Can you work these out from the model? Positions are in its coordinate system, mm. Face numbers are marked on the shaded views. A direction names the side the tool comes from. Give positions to 0.01 mm unless a question says otherwise; leave off trailing zeros. Loops run counter-clockwise (first coordinate to the right, second up) from the corner with the lowest first, then second, coordinate; pieces in that order, holes last. Notation, with made-up numbers: M 65.25,62 L 108.25,62 A29 cw 108.25,85 Z; hole C -22.75,20.25 d11. An arc over 180 degrees is marked long. Answer as a JSON object with one key per item and string values.
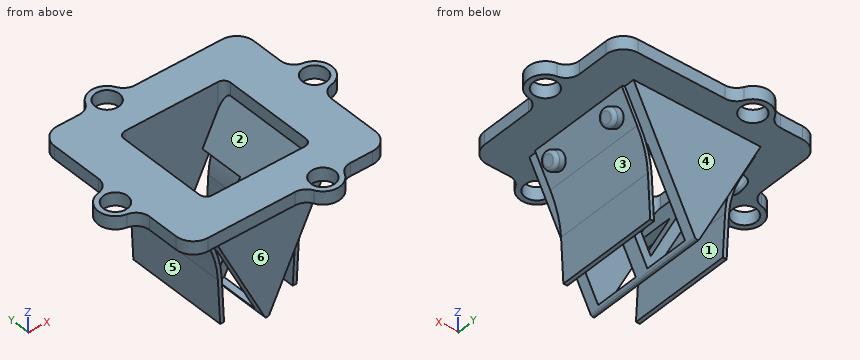
```python
from build123d import *

# Parameters (mm, degrees)
SKETCH_1_R          = 3.5
EXTRUDE_1_DEPTH     = 3.8
LOFT_START          = -18
LOFT_1_DEPTH        = 36
FILLET_1_R          = 0.5
CUT_EXTRUDE_1_DEPTH = 15
FILLET_2_R          = 2
SKETCH_6_W          = 22
SKETCH_6_H          = 13
CUT_EXTRUDE_2_DEPTH = 19
EXTRUDE_2_DEPTH     = 15
SKETCH_8_R          = 2.5
EXTRUDE_3_DEPTH     = 3
FILLET_5_R          = 1
SKETCH_9_R          = 2.5
EXTRUDE_4_DEPTH     = 3
FILLET_6_R          = 1


# Read off the part's stored shape, not the designer's step: По сечениям1
with BuildPart() as part:
    # Эскиз1 → Бобышка-Вытянуть1 (new body)
    with BuildSketch(Plane.XY):
        with BuildLine():
            Line((-24, -26), (1.437742252, -26))
            ThreePointArc((1.437742252, -26), (3.545927358, -26.600653658), (5.020967918, -28.222222222))
            ThreePointArc((5.020967918, -28.222222222), (9.5, -31), (13.979032082, -28.222222222))
            ThreePointArc((13.979032082, -28.222222222), (15.454072642, -26.600653658), (17.562257748, -26))
            Line((17.562257748, -26), (24, -26))
            ThreePointArc((24, -26), (27.535533906, -24.535533906), (29, -21))
            Line((29, -21), (29, -5.874119675))
            ThreePointArc((29, -5.874119675), (29.944949537, -3.292130777), (32.333333333, -1.930066486))
            ThreePointArc((32.333333333, -1.930066486), (36.5, 3), (32.333333333, 7.930066486))
            ThreePointArc((32.333333333, 7.930066486), (29.944949537, 9.292130777), (29, 11.874119675))
            Line((29, 11.874119675), (29, 21))
            ThreePointArc((29, 21), (27.535533906, 24.535533906), (24, 26))
            Line((24, 26), (-1.437742252, 26))
            ThreePointArc((-1.437742252, 26), (-3.545927358, 26.600653658), (-5.020967918, 28.222222222))
            ThreePointArc((-5.020967918, 28.222222222), (-9.5, 31), (-13.979032082, 28.222222222))
            ThreePointArc((-13.979032082, 28.222222222), (-15.454072642, 26.600653658), (-17.562257748, 26))
            Line((-17.562257748, 26), (-24, 26))
            ThreePointArc((-24, 26), (-27.535533906, 24.535533906), (-29, 21))
            Line((-29, 21), (-29, 5.874119675))
            ThreePointArc((-29, 5.874119675), (-29.944949537, 3.292130777), (-32.333333333, 1.930066486))
            ThreePointArc((-32.333333333, 1.930066486), (-36.5, -3), (-32.333333333, -7.930066486))
            ThreePointArc((-32.333333333, -7.930066486), (-29.944949537, -9.292130777), (-29, -11.874119675))
            Line((-29, -11.874119675), (-29, -21))
            ThreePointArc((-29, -21), (-27.535533906, -24.535533906), (-24, -26))
        make_face()
        with Locations(Location((31.5, 3, 0), (0, 0, 180))):
            Circle(SKETCH_1_R, mode=Mode.SUBTRACT)
        with Locations(Location((-9.5, 26, 0), (0, 0, 180))):
            Circle(SKETCH_1_R, mode=Mode.SUBTRACT)
        with Locations(Location((-31.5, -3, 0), (0, 0, 180))):
            Circle(SKETCH_1_R, mode=Mode.SUBTRACT)
        with Locations(Location((9.5, -26, 0), (0, 0, 180))):
            Circle(SKETCH_1_R, mode=Mode.SUBTRACT)
    extrude(amount=EXTRUDE_1_DEPTH)

    # По сечениям1 outline → По сечениям1 (add)
    with BuildSketch(Plane(origin=(0, 0, 0), x_dir=(1, 0, 0), z_dir=(0, 1, 0)).offset(LOFT_START)):
        Polygon((0.5, 36), (-0.5, 36), (-18.5, 0), (18.5, 0), align=None)
    extrude(amount=LOFT_1_DEPTH)

    # Скругление1
    fillet_1_edges = [part.edges().sort_by_distance(p)[0] for p in [
        (0.5, 0, -36),
        (-0.5, 0, -36),
    ]]
    fillet(fillet_1_edges, radius=FILLET_1_R)

    # Эскиз5 → Вырез-Вытянуть1 (cut, symmetric)
    with BuildSketch(Plane(origin=(0, 0, 0), x_dir=(1, 0, 0), z_dir=(0, 1, 0))):
        Polygon((15.5, -5.263726507), (-15.5, -5.263726507), (-15.5, 0), (0, 31), (15.5, 0), align=None)
    extrude(amount=CUT_EXTRUDE_1_DEPTH, both=True, mode=Mode.SUBTRACT)

    # Скругление2
    fillet_2_edges = [part.edges().sort_by_distance(p)[0] for p in [
        (15.5, -15, 1.9),
        (-15.5, -15, 1.9),
        (-15.5, 15, 1.9),
        (15.5, 15, 1.9),
    ]]
    fillet(fillet_2_edges, radius=FILLET_2_R)

    # Эскиз6 → Вырез-Вытянуть2 (cut, symmetric)
    with BuildSketch(Plane(origin=(0, 0, 0), x_dir=(0, 0, -1), z_dir=(1, 0, 0))):
        with Locations((24, 8.5)):
            Rectangle(SKETCH_6_W, SKETCH_6_H)
        with Locations((24, -8.5)):
            Rectangle(SKETCH_6_W, SKETCH_6_H)
    extrude(amount=CUT_EXTRUDE_2_DEPTH, both=True, mode=Mode.SUBTRACT)

    # Эскиз7 → Бобышка-Вытянуть2 (add, symmetric)
    with BuildSketch(Plane(origin=(0, 0, 0), x_dir=(1, 0, 0), z_dir=(0, 1, 0))):
        with BuildLine():
            Line((10, 34.139527531), (10.6733594, 21.251746752))
            ThreePointArc((10.6733594, 21.251746752), (11.624847718, 15.164834748), (13.799679679, 9.400640641))
            Line((13.799679679, 9.400640641), (18.5, 0))
            Line((18.5, 0), (19.394427191, 0.447213595))
            Line((19.394427191, 0.447213595), (14.917713668, 9.400640641))
            ThreePointArc((14.917713668, 9.400640641), (12.742881707, 15.164834748), (11.791393389, 21.251746752))
            Line((11.791393389, 21.251746752), (11.118033989, 34.139527531))
            Line((11.118033989, 34.139527531), (10, 34.139527531))
        make_face()
        with BuildLine():
            Line((-18.5, 0), (-19.394427191, 0.447213595))
            Line((-19.394427191, 0.447213595), (-14.917713668, 9.400640641))
            ThreePointArc((-14.917713668, 9.400640641), (-12.742881707, 15.164834748), (-11.791393389, 21.251746752))
            Line((-11.791393389, 21.251746752), (-11.118033989, 34.139527531))
            Line((-11.118033989, 34.139527531), (-10, 34.139527531))
            Line((-10, 34.139527531), (-10.6733594, 21.251746752))
            ThreePointArc((-10.6733594, 21.251746752), (-11.624847718, 15.164834748), (-13.799679679, 9.400640641))
            Line((-13.799679679, 9.400640641), (-18.5, 0))
        make_face()
    extrude(amount=EXTRUDE_2_DEPTH, both=True)

    # Эскиз8 → Бобышка-Вытянуть3 (add)
    with BuildSketch(Plane(origin=(15.694427191, 0, -7.847213595), x_dir=(-0.4472135954999576, 0, -0.8944271909999162), z_dir=(0.8944271909999162, 0, -0.4472135954999576))):
        with Locations(Location((-3, 10, 0), (0, 0, 180))):
            Circle(SKETCH_8_R)
        with Locations(Location((-3, -10, 0), (0, 0, 180))):
            Circle(SKETCH_8_R)
    extrude(amount=EXTRUDE_3_DEPTH)

    # Скругление5
    fillet_5_edges = [part.edges().sort_by_distance(p)[0] for p in [
        (18.601315562, 10, -8.741640786),
        (18.601315562, -10, -8.741640786),
    ]]
    fillet(fillet_5_edges, radius=FILLET_5_R)

    # Эскиз9 → Бобышка-Вытянуть4 (add)
    with BuildSketch(Plane(origin=(-15.694427191, 0, -7.847213595), x_dir=(-0.4472135954999576, 0, 0.8944271909999162), z_dir=(-0.8944271909999162, 0, -0.4472135954999576))):
        with Locations(Location((3, 10, 0), (0, 0, 180))):
            Circle(SKETCH_9_R)
        with Locations(Location((3, -10, 0), (0, 0, 180))):
            Circle(SKETCH_9_R)
    extrude(amount=EXTRUDE_4_DEPTH)

    # Скругление6
    fillet_6_edges = [part.edges().sort_by_distance(p)[0] for p in [
        (-20.837383539, 10, -4.269504832),
        (-20.837383539, -10, -4.269504832),
    ]]
    fillet(fillet_6_edges, radius=FILLET_6_R)


solid = part.part
```
1) Suppose I cut it at C-C, the plane z = -33. Write out the boundary of the cut face in (x, y), and give its area (3 significant figures).
Answer list:
{"outline": "M -11.18,-15 L -10.06,-15 L -10.06,15 L -11.18,15 Z; M -2,-18 L 2,-18 L 2,-15 L -2,-15 Z; M -2,-2 L 2,-2 L 2,2 L -2,2 Z; M -2,15 L 2,15 L 2,18 L -2,18 Z; M 10.06,-15 L 11.18,-15 L 11.18,15 L 10.06,15 Z", "area": "107 mm^2"}
2) If we mould it in two halves opening along Z, with no side actions, what happens to the marked faces 1, 2 and 3? For each: +Z half, -Z half, draft (parallel to the pull), parting line (faces both ways), or undercut.
Answer list:
{"face 1": "undercut", "face 2": "+Z half", "face 3": "-Z half"}
3) Please list where these lines run through material, in increasing order: line 1 along Y through (x, z) = (-9.5, 2.25); line 2 along Y through (x, z) = (9.5, 2.3); line 3 along X through (y, z) = (-1, -34). Write a range as from..to.
Answer list:
{"line 1": "-26..-15, 15..22.5, 29.5..31", "line 2": "-31..-29.5, -22.5..-15, 15..26", "line 3": "-11.13..-10.01, -1.5..1.5, 10.01..11.13"}
4) Suppose I cut it at A-A, the plane x = -2.5. Write out the boundary of the cut face in (y, z).
Answer list:
{"outline": "M -26,0 L -18,0 L -18,-32 L -15,-32 L -15,3.8 L -26,3.8 Z; M -2,-32 L 2,-32 L 2,-26 L -2,-26 Z; M 15,-32 L 18,-32 L 18,0 L 26.14,0 L 26.14,3.8 L 15,3.8 Z"}
5) Suppose I cut it at D-D, the plane x = 31.5. Write out the boundary of the cut face in (y, z), and give its area (3 significant figures).
Answer list:
{"outline": "M -2.17,0 L -0.5,0 L -0.5,3.8 L -2.17,3.8 Z; M 6.5,0 L 8.17,0 L 8.17,3.8 L 6.5,3.8 Z", "area": "12.7 mm^2"}
6) For the marked faces 4, 5 and 6, which set-ups out of +Z, -Z, +X, -X, +Y, -Y let a thin tool reach every point of the face, with its end or its side?
Answer list:
{"face 4": "-Z, +X, -X, +Y", "face 5": "-Z, -X, +Y, -Y", "face 6": "-Z, +X, -X, -Y"}
7) Will these pins go through, and if not, where does the flat tip stop? pin 1 Ø3 at (y, z) = (1.5, -2) entering from +X; pin 2 Ø0.9 at (x, y) = (10.5, 1.5) entering from -Z; pin 3 Ø11 at (x, z) = (-3, -13) entering from +Y; pin 4 Ø12 at (x, z) = (-19, -30) entering from +Y.
Answer list:
{"pin 1": "x = 19.37", "pin 2": "z = -34.14", "pin 3": "y = 18", "pin 4": "through"}
8) Suppose I cut it at B-B, the plane z = -17. Write out the boundary of the cut face in (x, y), and give its area (3 significant figures).
Answer list:
{"outline": "M -12.32,-15 L -11.2,-15 L -11.2,15 L -12.32,15 Z; M -10,-18 L 10,-18 L 10,-15 L -10,-15 Z; M -10,-2 L -7,-2 L -7,2 L -10,2 Z; M -10,15 L 10,15 L 10,18 L -10,18 Z; M 7,-2 L 10,-2 L 10,2 L 7,2 Z; M 11.2,-15 L 12.32,-15 L 12.32,15 L 11.2,15 Z", "area": "211 mm^2"}
